from build123d import *

# Parameters (mm, degrees)
SKETCH1_R               = 60
SKETCH1_R_2             = 2.25
SKETCH1_R_3             = 4
SKETCH1_R_4             = 1.5
SKETCH1_W               = 22.2
SKETCH1_H               = 40.9
BOSS_EXTRUDE1_DEPTH     = 2
SKETCH2_W               = 3
SKETCH2_H               = 10
CUT_EXTRUDE_THIN1_DEPTH = 85.876380696


with BuildPart() as part:
    # Sketch1 → Boss-Extrude1 (new body)
    with BuildSketch(Plane(origin=(0, 0, 0), x_dir=(1, 0, 0), z_dir=(0, 1, 0))):
        with Locations(Location((0, 0, 0), (0, 0, 270))):
            Circle(SKETCH1_R)
        with Locations(Location((0, 50, 0), (0, 0, 270))):
            Circle(SKETCH1_R_2, mode=Mode.SUBTRACT)
        with Locations(Location((50, 0, 0), (0, 0, 270))):
            Circle(SKETCH1_R_2, mode=Mode.SUBTRACT)
        with Locations(Location((0, -50, 0), (0, 0, 270))):
            Circle(SKETCH1_R_2, mode=Mode.SUBTRACT)
        with Locations(Location((-50, 0, 0), (0, 0, 270))):
            Circle(SKETCH1_R_2, mode=Mode.SUBTRACT)
        with Locations(Location((-4.932420963, 35.45, 0), (0, 0, 270))):
            Circle(SKETCH1_R_2, mode=Mode.SUBTRACT)
        with Locations(Location((5.067579037, 35.45, 0), (0, 0, 270))):
            Circle(SKETCH1_R_2, mode=Mode.SUBTRACT)
        with Locations(Location((5.067579037, -14.55, 0), (0, 0, 270))):
            Circle(SKETCH1_R_2, mode=Mode.SUBTRACT)
        with Locations(Location((-4.932420963, -14.55, 0), (0, 0, 270))):
            Circle(SKETCH1_R_2, mode=Mode.SUBTRACT)
        with Locations(Location((-35, 0, 0), (0, 0, 270))):
            Circle(SKETCH1_R_3, mode=Mode.SUBTRACT)
        with Locations(Location((-42.5, 0, 0), (0, 0, 270))):
            Circle(SKETCH1_R_4, mode=Mode.SUBTRACT)
        with Locations(Location((-35, 7.5, 0), (0, 0, 270))):
            Circle(SKETCH1_R_4, mode=Mode.SUBTRACT)
        with Locations(Location((-27.5, 0, 0), (0, 0, 270))):
            Circle(SKETCH1_R_4, mode=Mode.SUBTRACT)
        with Locations(Location((-35, -7.5, 0), (0, 0, 270))):
            Circle(SKETCH1_R_4, mode=Mode.SUBTRACT)
        with Locations(Location((42.5, 0, 0), (0, 0, 270))):
            Circle(SKETCH1_R_4, mode=Mode.SUBTRACT)
        with Locations(Location((35, 0, 0), (0, 0, 270))):
            Circle(SKETCH1_R_3, mode=Mode.SUBTRACT)
        with Locations(Location((35, -7.5, 0), (0, 0, 270))):
            Circle(SKETCH1_R_4, mode=Mode.SUBTRACT)
        with Locations(Location((27.5, 0, 0), (0, 0, 270))):
            Circle(SKETCH1_R_4, mode=Mode.SUBTRACT)
        with Locations(Location((35, 7.5, 0), (0, 0, 270))):
            Circle(SKETCH1_R_4, mode=Mode.SUBTRACT)
        with Locations((0.067579037, 10.45)):
            Rectangle(SKETCH1_W, SKETCH1_H, mode=Mode.SUBTRACT)
    extrude(amount=BOSS_EXTRUDE1_DEPTH)

    # Sketch2 → Cut-Extrude-Thin1 (cut, through all)
    with BuildSketch(Plane.XZ):
        with Locations((0.067579037, 15)):
            Rectangle(SKETCH2_W, SKETCH2_H)
        with Locations((0.067579037, -35.9)):
            Rectangle(SKETCH2_W, SKETCH2_H)
    extrude(amount=-CUT_EXTRUDE_THIN1_DEPTH, mode=Mode.SUBTRACT)


solid = part.part
For this review, take the finished solid that the model builds, in its own axes (mm). Coordinates: 2 decimals unless noted, no trailing zeros. Order: outer loops, then holes, each group sorted by start corner. A loop starts at its lowest first (then second) coordinate and runs counter-clockwise, first axis right, second up. Notation, with made-up numbers: (83.25, 39.5) - (135.25, 39.5) arc R20 ccw to (135.25, 46.5) - close; hole circle Ø9 at (46, -5). An arc over 180 degrees is marked (long way). Answer as CSV lines item,"result". Start each with the question number.
1) Draft analysis for pull direction Z (two halves, no side actions). For faces 1 (the cylindrical face through (2.64, 0.99, -59.94)), 2 (the flat face through (-12, 2, -1)), 3 (the cylindrical face through (0.099, 0.986, 47.752)), state which applies: +Z half, -Z half, draft (parallel to the pull), parting line (faces both ways), or undercut.
2) Add section D-D (x = -50). State the section outline as (y, z) points.
3) Add section B-B (z = 49.5). State the section outline as (x, y) points.
4) Add section A-A (z = -35.45). State the section outline as (x, y) points.
5) To check wall thickness, follow line 1 along X through (y, z) = (1.8, -23); line 2 along X through (y, z) = (1.4, 50); line 3 along X through (y, z) = (1.65, -36). State the ranges of each line that lie inside material, in increasing order. Write a range as [from, to].
6) Add section C-C (x = 35). State the section outline as (y, z) points, then the cut area to 3 significant figures.
7) Insertion check: P1, Ø2.5, axis at x = 27.5, z = 0, coming from the +Y side; P2, Ø0.6, axis at y = 1, z = -35, coming from the -X side. Each pin has a flat end and moves straight along its axis. Give the tip position at first contact, or say it passes through.
Result:
1,face 1,"parting line"
1,face 2,"draft"
1,face 3,"undercut"
2,outline,"(0, -33.17) - (2, -33.17) - (2, -2.25) - (0, -2.25) - close; (0, 2.25) - (2, 2.25) - (2, 33.17) - (0, 33.17) - close"
3,outline,"(-33.91, 0) - (-2.19, 0) - (-2.19, 2) - (-33.91, 2) - close; (2.19, 0) - (33.91, 0) - (33.91, 2) - (2.19, 2) - close"
4,outline,"(-48.41, 0) - (-7.18, 0) - (-7.18, 2) - (-48.41, 2) - close; (-2.68, 0) - (-1.43, 0) - (-1.43, 2) - (-2.68, 2) - close; (1.57, 0) - (2.82, 0) - (2.82, 2) - (1.57, 2) - close; (7.32, 0) - (48.41, 0) - (48.41, 2) - (7.32, 2) - close"
5,line 1,"[-55.42, -11.03], [11.17, 55.42]"
5,line 2,"[-33.17, -2.25], [2.25, 33.17]"
5,line 3,"[-48, -7.11], [-2.75, -1.43], [1.57, 2.89], [7.25, 48]"
6,outline,"(0, -48.73) - (2, -48.73) - (2, -9) - (0, -9) - close; (0, -6) - (2, -6) - (2, -4) - (0, -4) - close; (0, 4) - (2, 4) - (2, 6) - (0, 6) - close; (0, 9) - (2, 9) - (2, 48.73) - (0, 48.73) - close"
6,area,"167 mm^2"
7,P1,"through"
7,P2,"x = -48.95"
